```python
from build123d import *

# Parameters (mm, degrees)
BOSS_EXTRUDE1_DEPTH  = 118
SKETCH2_W            = 68
SKETCH2_H            = 10
BOSS_EXTRUDE2_DEPTH  = 12
SKETCH4_W            = 2
SKETCH4_H            = 5.241203994
BOSS_EXTRUDE4_DEPTH  = 118
SKETCH5_W            = 40
SKETCH5_H            = 14
CUT_EXTRUDE1_DEPTH   = 12
BOSS_EXTRUDE5_START  = -2
SKETCH6_W            = 0.5
SKETCH6_H            = 14
BOSS_EXTRUDE5_DEPTH  = 2
SKETCH7_W            = 118
SKETCH7_H            = 2
BOSS_EXTRUDE6_DEPTH  = 2
SKETCH8_W            = 2
SKETCH8_H            = 0.649840642
BOSS_EXTRUDE7_DEPTH  = 50
BOSS_EXTRUDE8_DEPTH  = 2
SKETCH11_W           = 222
SKETCH11_H           = 2
BOSS_EXTRUDE9_DEPTH  = 2
SKETCH13_W           = 118
SKETCH13_H           = 2
BOSS_EXTRUDE10_DEPTH = 4
SKETCH14_W           = 1
SKETCH14_H           = 46
CUT_EXTRUDE2_DEPTH   = 4
SKETCH15_W           = 215
SKETCH15_H           = 1
CUT_EXTRUDE3_DEPTH   = 4
SKETCH16_W           = 215
SKETCH16_H           = 1
CUT_EXTRUDE4_DEPTH   = 4
SKETCH17_W           = 155.2
SKETCH17_H           = 87.1
CUT_EXTRUDE5_DEPTH   = 4
SKETCH18_W           = 175.2
SKETCH18_H           = 97.1
BOSS_EXTRUDE11_DEPTH = 1
SKETCH19_W           = 155.2
SKETCH19_H           = 87.1
CUT_EXTRUDE6_DEPTH   = 1
SKETCH20_R           = 1.5
CUT_EXTRUDE7_DEPTH   = 47.46373967
SKETCH21_W           = 80
SKETCH21_H           = 10
BOSS_EXTRUDE12_DEPTH = 12
SKETCH22_W           = 80
SKETCH22_H           = 5
CUT_EXTRUDE8_DEPTH   = 12
SKETCH23_W           = 10
SKETCH23_H           = 10
BOSS_EXTRUDE13_DEPTH = 12
BOSS_EXTRUDE14_START = -10
SKETCH24_W           = 12
SKETCH24_H           = 4
BOSS_EXTRUDE14_DEPTH = 10
BOSS_EXTRUDE15_START = -10
SKETCH25_W           = 8
SKETCH25_H           = 1
BOSS_EXTRUDE15_DEPTH = 10
SKETCH27_W           = 80
SKETCH27_H           = 10
BOSS_EXTRUDE16_DEPTH = 5
BOSS_EXTRUDE17_DEPTH = 2
SKETCH30_W           = 80
SKETCH30_H           = 10
BOSS_EXTRUDE18_DEPTH = 10
SKETCH31_W           = 50
SKETCH31_H           = 11.87067785
BOSS_EXTRUDE20_DEPTH = 10
SKETCH32_W           = 50
SKETCH32_H           = 1.87
CUT_EXTRUDE9_DEPTH   = 10


with BuildPart() as part:
    # Sketch1 → Boss-Extrude1 (new body)
    with BuildSketch(Plane.XY):
        Polygon((94.417554234, -32.563143832), (94.417554234, 17.436856168), (-87.582445766, 62.195652174), (-127.582445766, 62.195652174), (-127.582445766, -37.804347826), (-125.582445766, -37.757129772), (-125.582445766, 60.242870228), (-88.016763075, 60.242870228), (92.417554234, 15.869118575), (92.417554234, 15.389638114), (92.417554234, -32.610361886), align=None)
    extrude(amount=BOSS_EXTRUDE1_DEPTH)

    # Sketch2 → Boss-Extrude2 (add)
    with BuildSketch(Plane.ZY.offset(127.582445766)):
        with Locations((84, -32.804347826)):
            Rectangle(SKETCH2_W, SKETCH2_H)
    extrude(amount=-BOSS_EXTRUDE2_DEPTH)

    # Sketch4 → Boss-Extrude4 (add)
    with BuildSketch(Plane.XY.offset(118)):
        with Locations((93.417554234, -35.183745829)):
            Rectangle(SKETCH4_W, SKETCH4_H)
    extrude(amount=-BOSS_EXTRUDE4_DEPTH)

    # Sketch5 → Cut-Extrude1 (cut)
    with BuildSketch(Plane(origin=(94.417554234, 0, 0), x_dir=(0, 0, -1), z_dir=(1, 0, 0))):
        with Locations((-29.5, -27.304347826)):
            Rectangle(SKETCH5_W, SKETCH5_H)
    extrude(amount=-CUT_EXTRUDE1_DEPTH, mode=Mode.SUBTRACT)

    # Sketch6 → Boss-Extrude5 (add)
    with BuildSketch(Plane(origin=(94.417554234, 0, 0), x_dir=(0, 0, -1), z_dir=(1, 0, 0)).offset(BOSS_EXTRUDE5_START)):
        with Locations((-49.25, -27.304347826)):
            Rectangle(SKETCH6_W, SKETCH6_H)
    extrude(amount=BOSS_EXTRUDE5_DEPTH)

    # Sketch7 → Boss-Extrude6 (add)
    with BuildSketch(Plane.ZY.offset(-92.417554234)):
        with Locations((59, -36.804347826)):
            Rectangle(SKETCH7_W, SKETCH7_H)
    extrude(amount=BOSS_EXTRUDE6_DEPTH)

    # Sketch8 → Boss-Extrude7 (add)
    with BuildSketch(Plane(origin=(0, 0, 50), x_dir=(-1, 0, 0), z_dir=(0, 0, -1))):
        with Locations((126.582445766, -37.479427505)):
            Rectangle(SKETCH8_W, SKETCH8_H)
    extrude(amount=BOSS_EXTRUDE7_DEPTH)

    # Sketch10 → Boss-Extrude8 (add)
    with BuildSketch(Plane(origin=(0, 0, 0), x_dir=(-1, 0, 0), z_dir=(0, 0, -1))):
        Polygon((-94.417554234, 17.436856168), (87.582445766, 62.195652174), (127.582445766, 62.195652174), (127.582445766, -37.804347826), (-94.417554234, -37.804347826), align=None)
    extrude(amount=-BOSS_EXTRUDE8_DEPTH)

    # Sketch11 → Boss-Extrude9 (add)
    with BuildSketch(Plane.XY.offset(2)):
        with Locations((-16.582445766, -36.804347826)):
            Rectangle(SKETCH11_W, SKETCH11_H)
    extrude(amount=BOSS_EXTRUDE9_DEPTH)

    # Sketch13 → Boss-Extrude10 (add)
    with BuildSketch(Plane.ZY.offset(127.582445766)):
        with Locations((59, -36.804347826)):
            Rectangle(SKETCH13_W, SKETCH13_H)
    extrude(amount=-BOSS_EXTRUDE10_DEPTH)

    # Sketch14 → Cut-Extrude2 (cut)
    with BuildSketch(Plane(origin=(0, -35.804347826, 0), x_dir=(1, 0, 0), z_dir=(0, 1, 0))):
        with Locations((-124.082445766, -27)):
            Rectangle(SKETCH14_W, SKETCH14_H)
    extrude(amount=-CUT_EXTRUDE2_DEPTH, mode=Mode.SUBTRACT)

    # Sketch15 → Cut-Extrude3 (cut)
    with BuildSketch(Plane.XZ.offset(37.804347826)):
        with Locations((-17.082445766, 3.5)):
            Rectangle(SKETCH15_W, SKETCH15_H)
    extrude(amount=-CUT_EXTRUDE3_DEPTH, mode=Mode.SUBTRACT)

    # Sketch16 → Cut-Extrude4 (cut)
    with BuildSketch(Plane.XZ.offset(37.804347826)):
        with Locations((-17.082445766, 2.5)):
            Rectangle(SKETCH16_W, SKETCH16_H)
    extrude(amount=-CUT_EXTRUDE4_DEPTH, mode=Mode.SUBTRACT)

    # Sketch17 → Cut-Extrude5 (cut)
    with BuildSketch(Plane(origin=(9.428373652, 38.338028676, 0), x_dir=(0.971065881, -0.238811756, 0), z_dir=(0.238811756, 0.971065881, 0))):
        with Locations((-6.191377784, -59)):
            Rectangle(SKETCH17_W, SKETCH17_H)
    extrude(amount=-CUT_EXTRUDE5_DEPTH, mode=Mode.SUBTRACT)

    # Sketch18 → Boss-Extrude11 (add)
    with BuildSketch(Plane(origin=(8.95075014, 36.395896914, 0), x_dir=(0.971065881, -0.238811756, 0), z_dir=(-0.238811756, -0.971065881, 0))):
        with Locations((-6.191377784, 59)):
            Rectangle(SKETCH18_W, SKETCH18_H)
    extrude(amount=BOSS_EXTRUDE11_DEPTH)

    # Sketch19 → Cut-Extrude6 (cut)
    with BuildSketch(Plane(origin=(8.95075014, 36.395896914, 0), x_dir=(0.971065881, -0.238811756, 0), z_dir=(0.238811756, 0.971065881, 0))):
        with Locations((-6.191377784, -59)):
            Rectangle(SKETCH19_W, SKETCH19_H)
    extrude(amount=-CUT_EXTRUDE6_DEPTH, mode=Mode.SUBTRACT)

    # Sketch20 → Cut-Extrude7 (cut, through all)
    with BuildSketch(Plane(origin=(8.711938383, 35.424831033, 0), x_dir=(0.971065881, -0.238811756, 0), z_dir=(-0.238811756, -0.971065881, 0))):
        with Locations((-88.791377784, 92.55)):
            Circle(SKETCH20_R)
        with Locations((-88.791377784, 25.45)):
            Circle(SKETCH20_R)
        with Locations((76.408622216, 25.45)):
            Circle(SKETCH20_R)
        with Locations((76.408622216, 92.55)):
            Circle(SKETCH20_R)
    extrude(amount=-CUT_EXTRUDE7_DEPTH, mode=Mode.SUBTRACT)

    # Sketch21 → Boss-Extrude12 (add)
    with BuildSketch(Plane(origin=(0, 0, 0), x_dir=(-1, 0, 0), z_dir=(0, 0, -1))):
        with Locations((60.582445766, -32.804347826)):
            Rectangle(SKETCH21_W, SKETCH21_H)
    extrude(amount=-BOSS_EXTRUDE12_DEPTH)

    # Sketch22 → Cut-Extrude8 (cut)
    with BuildSketch(Plane.XZ.offset(37.804347826)):
        with Locations((-60.582445766, 9.5)):
            Rectangle(SKETCH22_W, SKETCH22_H)
    extrude(amount=-CUT_EXTRUDE8_DEPTH, mode=Mode.SUBTRACT)

    # Sketch23 → Boss-Extrude13 (add)
    with BuildSketch(Plane(origin=(94.417554234, 0, 0), x_dir=(0, 0, -1), z_dir=(1, 0, 0))):
        with Locations((-61, -32.804347826)):
            Rectangle(SKETCH23_W, SKETCH23_H)
    extrude(amount=-BOSS_EXTRUDE13_DEPTH)

    # Sketch24 → Boss-Extrude14 (add)
    with BuildSketch(Plane.XZ.offset(37.804347826).offset(BOSS_EXTRUDE14_START)):
        with Locations((88.417554234, 54)):
            Rectangle(SKETCH24_W, SKETCH24_H)
    extrude(amount=BOSS_EXTRUDE14_DEPTH)

    # Sketch25 → Boss-Extrude15 (add)
    with BuildSketch(Plane.XZ.offset(37.804347826).offset(BOSS_EXTRUDE15_START)):
        with Locations((86.417554234, 51.5)):
            Rectangle(SKETCH25_W, SKETCH25_H)
    extrude(amount=BOSS_EXTRUDE15_DEPTH)

    # Sketch27 → Boss-Extrude16 (add)
    with BuildSketch(Plane.XY.offset(2)):
        with Locations((28.917554234, -32.804347826)):
            Rectangle(SKETCH27_W, SKETCH27_H)
    extrude(amount=BOSS_EXTRUDE16_DEPTH)

    # Sketch28 → Boss-Extrude17 (add)
    with BuildSketch(Plane.XY.offset(118)):
        Polygon((-127.582445766, -37.804347826), (94.417554234, -37.804347826), (94.417554234, 17.436856168), (-87.582445766, 62.195652174), (-127.582445766, 62.195652174), align=None)
    extrude(amount=BOSS_EXTRUDE17_DEPTH)

    # Sketch30 → Boss-Extrude18 (add)
    with BuildSketch(Plane.XZ.offset(37.804347826)):
        with Locations((-60.582445766, 113)):
            Rectangle(SKETCH30_W, SKETCH30_H)
    extrude(amount=-BOSS_EXTRUDE18_DEPTH)

    # Sketch31 → Boss-Extrude20 (add)
    with BuildSketch(Plane(origin=(0, 0, 118), x_dir=(-1, 0, 0), z_dir=(0, 0, -1))):
        with Locations((-14.417554234, -31.869008901)):
            Rectangle(SKETCH31_W, SKETCH31_H)
    extrude(amount=BOSS_EXTRUDE20_DEPTH)

    # Sketch32 → Cut-Extrude9 (cut)
    with BuildSketch(Plane(origin=(0, 0, 108), x_dir=(-1, 0, 0), z_dir=(0, 0, -1))):
        with Locations((-14.417554234, -26.868669976)):
            Rectangle(SKETCH32_W, SKETCH32_H)
    extrude(amount=-CUT_EXTRUDE9_DEPTH, mode=Mode.SUBTRACT)


solid = part.part
```
CAD build for the part. Positions are in the model's coordinates, mm. A direction names the side the tool comes from. Round coordinates to 2 decimals unless told otherwise and drop trailing zeros. Write each loop counter-clockwise with the first axis right and the second up, starting at its lowest first coordinate (ties: lowest second). Pieces come first, ordered by that corner, then holes.
Item 1: Tool access for faces 1 (the flat face through (-61, -33, 108)), 2 (the flat face through (-107, 60.243, 59)), 3 (the flat face through (-42, -37.804, 109)): list every direction of +Z, -Z, +X, -X, +Y, -Y with a clear straight run to the whole face (end or side of a thin tool).
Filled in:
face 1: -Y
face 2: none
face 3: +Z, -Z, +X, -X, -Y
Item 2: Band-saw the part on C-C on z = 111. Write the cut outline in (x, y).
Filled in:
outline: (-127.58, -37.8) - (-115.58, -37.8) - (-115.58, -27.8) - (-125.58, -27.8) - (-125.58, 60.24) - (-88.02, 60.24) - (92.42, 15.87) - (92.42, -35.8) - (90.42, -35.8) - (90.42, -37.8) - (94.42, -37.8) - (94.42, 17.44) - (-87.58, 62.2) - (-127.58, 62.2) - close; (-100.58, -37.8) - (-20.58, -37.8) - (-20.58, -27.8) - (-100.58, -27.8) - close; (-10.58, -37.8) - (39.42, -37.8) - (39.42, -27.8) - (-10.58, -27.8) - close
Item 3: Band-saw the part on D-D on x = 43.5. Write the cut outline in (y, z).
Filled in:
outline: (-37.8, 0) - (29.96, 0) - (29.96, 15.45) - (26.87, 15.45) - (26.87, 10.45) - (27.9, 10.45) - (27.9, 2) - (-27.8, 2) - (-27.8, 7) - (-37.8, 7) - close; (-37.8, 118) - (27.9, 118) - (27.9, 107.55) - (26.87, 107.55) - (26.87, 102.55) - (29.96, 102.55) - (29.96, 120) - (-37.8, 120) - close
Item 4: Drill centre lines: L1, parallel to Z at x = -76, y = -27; L2, parallel to X at y = 13, z = 84; L3, parallel to X at y = -28.5, z = 54. Where is each one in solid material? Low to high.
Filled in:
L1: z = 0 to 2, 118 to 120
L2: x = -127.58 to -125.58, 92.42 to 94.42
L3: x = -127.58 to -115.58, 82.42 to 94.42
Item 5: Band-saw the part on B-B on y = -10. Write the cut outline in (x, z).
Filled in:
outline: (-127.58, 0) - (94.42, 0) - (94.42, 120) - (-127.58, 120) - close; hole (-125.58, 2) - (92.42, 2) - (92.42, 118) - (-125.58, 118) - close
Item 6: Mould opens along X. For faces 4 (the flat face through (-15, 2, 0)), 5 (the flat face through (-100.582, -33, 4)), 6 (the flat face through (-127.582, 13, 59)) say: released by +X, released by -X, zero draft, split by the parting line, or undercut.
Filled in:
face 4: zero draft
face 5: undercut
face 6: released by -X
Item 7: Band-saw the part on A-A on z = 68.5. Write the cut outline in (x, y) (1 decimal).
Filled in:
outline: (-127.6, -37.8) - (-115.6, -37.8) - (-115.6, -27.8) - (-125.6, -27.8) - (-125.6, 60.2) - (-88, 60.2) - (-82.1, 58.8) - (-82.4, 57.8) - (-72.7, 55.4) - (-71.9, 58.3) - (-87.6, 62.2) - (-127.6, 62.2) - close; (78.1, 18.4) - (87.8, 16) - (88, 17) - (92.4, 15.9) - (92.4, -35.8) - (90.4, -35.8) - (90.4, -37.8) - (94.4, -37.8) - (94.4, 17.4) - (78.8, 21.3) - close
Item 8: Drop flat-ended pins along their axis: pin 1 Ø8 at (x, y) = (-70.5, -30.5) entering from -Z; pin 2 Ø3 at (x, z) = (18.5, 111.5) entering from +Y; pin 3 Ø4 at (x, z) = (33.5, 3.5) entering from +Y; pin 4 Ø3 at (x, z) = (-47.5, 115) entering from +Y. Give the stop position or say it passes through.
Filled in:
pin 1: stops at z = 0
pin 2: stops at y = 36.48
pin 3: stops at y = 32.91
pin 4: stops at y = 52.71
